For this review, take the finished solid that the model builds, in its own axes (mm). A direction names the side the tool comes from. Round coordinates to 2 decimals unless told otherwise and drop trailing zeros. Write each loop counter-clockwise with the first axis right and the second up, starting at its lowest first coordinate (ties: lowest second). Pieces come first, ordered by that corner, then holes.
from build123d import *

# Parameters (mm, degrees)
SUPPORTOMOTORE_DEPTH     = 30
SCHIZZO2_W               = 58
SCHIZZO2_H               = 39
SUPPORTOESC_DEPTH        = 4
COLONNESUPPORTOESC_REACH = 62.166
SCHIZZO3_R               = 3
SCHIZZO7_W               = 5
SCHIZZO7_H               = 5
SUPPORTIBASEMOTORE_DEPTH = 15
SCHIZZO8_W               = 30
SCHIZZO8_H               = 30
BASEMOTORE_DEPTH         = 2
SCHIZZO9_R               = 1.5
SCHIZZO9_R_2             = 4
FORIAGGANCIOMOTORE_DEPTH = 2
SCHIZZO10_W              = 20
SCHIZZO10_H              = 4
APERTURAFASCETTA_DEPTH   = 4


with BuildPart() as part:
    # Schizzo1 → SupportoMotore (new body)
    with BuildSketch(Plane.XY):
        with BuildLine():
            Line((-2.5, -10.712142643), (-2.5, -15.712142643))
            Line((-2.5, -15.712142643), (-7.5, -15.712142643))
            Line((-7.5, -15.712142643), (-7.5, -8.04673847))
            ThreePointArc((-7.5, -8.04673847), (-10.999946955, -0.034161219), (-7.549834435, 8))
            Line((-7.549834435, 8), (-15.935446939, 8))
            Line((-15.935446939, 8), (-15.935446939, 11))
            Line((-15.935446939, 11), (14.064553061, 11))
            Line((14.064553061, 11), (14.064553061, 8))
            Line((14.064553061, 8), (7.549834435, 8))
            ThreePointArc((7.549834435, 8), (10.999946955, -0.034161219), (7.5, -8.04673847))
            Line((7.5, -8.04673847), (7.5, -15.712142643))
            Line((7.5, -15.712142643), (2.5, -15.712142643))
            Line((2.5, -15.712142643), (2.5, -10.712142643))
            Line((2.5, -10.712142643), (2.5, -8.645808233))
            ThreePointArc((2.5, -8.645808233), (0, 9), (-2.5, -8.645808233))
            Line((-2.5, -8.645808233), (-2.5, -10.712142643))
        make_face()
    extrude(amount=SUPPORTOMOTORE_DEPTH)

    # Schizzo2 → SupportoESC (add)
    with BuildSketch(Plane(origin=(14.064553061, 0, 0), x_dir=(0, 0, -1), z_dir=(1, 0, 0))):
        with Locations((-15, -8.5)):
            Rectangle(SCHIZZO2_W, SCHIZZO2_H)
    extrude(amount=SUPPORTOESC_DEPTH)

    # Schizzo3 → ColonneSupportoESC (add, up to next)
    with BuildSketch(Plane.ZY.offset(-14.064553061), mode=Mode.PRIVATE) as colonnesupportoesc_sk1:
        with Locations(Location((22, -6, 0), (0, 0, 223.019415965))):
            Circle(SCHIZZO3_R)
    colonnesupportoesc_tool1 = extrude(colonnesupportoesc_sk1.sketch, amount=COLONNESUPPORTOESC_REACH, mode=Mode.PRIVATE) - part.part
    # Schizzo3 → ColonneSupportoESC (add, up to next)
    with BuildSketch(Plane.ZY.offset(-14.064553061), mode=Mode.PRIVATE) as colonnesupportoesc_sk2:
        with Locations(Location((8, -6, 0), (0, 0, 223.019415965))):
            Circle(SCHIZZO3_R)
    colonnesupportoesc_tool2 = extrude(colonnesupportoesc_sk2.sketch, amount=COLONNESUPPORTOESC_REACH, mode=Mode.PRIVATE) - part.part
    add(colonnesupportoesc_tool1.solids().sort_by_distance((14.064553, -6, 22))[0])
    add(colonnesupportoesc_tool2.solids().sort_by_distance((14.064553, -6, 8))[0])

    # Schizzo7 → SupportiBaseMotore (add)
    with BuildSketch(Plane(origin=(0, 11, 0), x_dir=(1, 0, 0), z_dir=(0, 1, 0))):
        with Locations((-13.435446939, -27.5)):
            Rectangle(SCHIZZO7_W, SCHIZZO7_H)
        with Locations((11.564553061, -27.5)):
            Rectangle(SCHIZZO7_W, SCHIZZO7_H)
        with Locations((11.564553061, -2.5)):
            Rectangle(SCHIZZO7_W, SCHIZZO7_H)
        with Locations((-13.435446939, -2.5)):
            Rectangle(SCHIZZO7_W, SCHIZZO7_H)
    extrude(amount=SUPPORTIBASEMOTORE_DEPTH)

    # Schizzo8 → BaseMotore (add)
    with BuildSketch(Plane(origin=(0, 26, 0), x_dir=(1, 0, 0), z_dir=(0, 1, 0))):
        with Locations((-0.935446939, -15)):
            Rectangle(SCHIZZO8_W, SCHIZZO8_H)
    extrude(amount=BASEMOTORE_DEPTH)

    # Schizzo9 → ForiAggancioMotore (cut)
    with BuildSketch(Plane(origin=(0, 28, 0), x_dir=(1, 0, 0), z_dir=(0, 1, 0))):
        with Locations(Location((2.623315698, -23.808246618, 0), (0, 0, 270))):
            Circle(SCHIZZO9_R)
        with Locations(Location((-9.743693557, -18.558762637, 0), (0, 0, 270))):
            Circle(SCHIZZO9_R)
        with Locations(Location((-4.494209576, -6.191753382, 0), (0, 0, 270))):
            Circle(SCHIZZO9_R)
        with Locations(Location((7.872799679, -11.441237363, 0), (0, 0, 270))):
            Circle(SCHIZZO9_R)
        with Locations(Location((-0.935446939, -15, 0), (0, 0, 270))):
            Circle(SCHIZZO9_R_2)
    extrude(amount=-FORIAGGANCIOMOTORE_DEPTH, mode=Mode.SUBTRACT)

    # Schizzo10 → AperturaFascetta (cut)
    with BuildSketch(Plane(origin=(18.064553061, 0, 0), x_dir=(0, 0, -1), z_dir=(1, 0, 0))):
        with Locations((-15, 6)):
            Rectangle(SCHIZZO10_W, SCHIZZO10_H)
        with Locations((-15, -23)):
            Rectangle(SCHIZZO10_W, SCHIZZO10_H)
    extrude(amount=-APERTURAFASCETTA_DEPTH, mode=Mode.SUBTRACT)


solid = part.part
(1) We need section A-A, the plane y = 16.5. Give the boundary of the cut face in (x, z).
Geometry check:
outline: (-15.94, 0) - (-10.94, 0) - (-10.94, 5) - (-15.94, 5) - close; (-15.94, 25) - (-10.94, 25) - (-10.94, 30) - (-15.94, 30) - close; (9.06, 0) - (14.06, 0) - (14.06, 5) - (9.06, 5) - close; (9.06, 25) - (14.06, 25) - (14.06, 30) - (9.06, 30) - close
(2) For pin 1 Ø1 at (y, z) = (-9, 4) entering from -X; pin 2 Ø5.5 at (x, z) = (4.5, 11.5) entering from -Y; pin 3 Ø5.5 at (x, z) = (11, 8) entering from -Y, all flat-tipped, find the tip position at first contact; note any pin that passes through.
Geometry check:
pin 1: stops at x = -7.5
pin 2: stops at y = -15.71
pin 3: stops at y = -9
(3) We need section D-D, the plane z = 15. State how many separate pieces and enclosed holes the cut face has, and give its area (3 significant figures).
Geometry check:
separate pieces: 5
enclosed holes: 0
area: 403 mm2
(4) Mouldability with a two-part tool opening along X and no side actions: class faces 1 (the face through (-15.935, 17.9, 25.2)), 2 (the face through (11.56, -8.95, 8.55)), 3 (the face through (16, -21, 15)) as pulls with the +X half, pulls with the -X half, needs draft (parallel to the pull), parting line crosses it, or undercut.
Geometry check:
face 1: pulls with the -X half
face 2: undercut
face 3: needs draft
(5) We need section B-B, the plane z = 27. Give the boundary of the cut face in (x, y).
Geometry check:
outline: (-15.94, 8) - (-7.55, 8) arc R11 ccw to (-7.5, -8.05) - (-7.5, -15.71) - (-2.5, -15.71) - (-2.5, -8.65) arc R9 cw (long way) to (2.5, -8.65) - (2.5, -15.71) - (7.5, -15.71) - (7.5, -8.05) arc R11 ccw to (7.55, 8) - (14.06, 8) - (14.06, -28) - (18.06, -28) - (18.06, 11) - (14.06, 11) - (14.06, 28) - (-15.94, 28) - close; hole (-10.94, 11) - (9.06, 11) - (9.06, 26) - (-10.94, 26) - close
(6) For line 1 along Y through (x, z) = (5, 17); line 2 along Y through (x, z) = (-11.5, 20); line 3 along Y through (x, z) = (16, 21), list the stretches that pass through material, from the lowest coordinate up.
Geometry check:
line 1: y = -15.71 to -7.48, 7.48 to 11, 26 to 28
line 2: y = 8 to 11, 26 to 28
line 3: y = -28 to -25, -21 to 4, 8 to 11
(7) For faces 4 (the face through (-10.935, 18, 3)), 5 (the face through (5, -15.712, 15)), 6 (the face through (-12, 8, 15)), list the 3-axis set-ups (+Z, -Z, +X, -X, +Y, -Y) from which the entire face can be reached by the end or side of a thin tool; tool diameter is ignored.
Geometry check:
face 4: +Z, -Z
face 5: +Z, -Z, -X, -Y
face 6: +Z, -Z, -X
(8) We need section C-C, the plane y = -10. Give the boundary of the cut face in (x, z), and give its area (3 significant figures).
Geometry check:
outline: (-7.5, 0) - (-2.5, 0) - (-2.5, 30) - (-7.5, 30) - close; (2.5, 0) - (7.5, 0) - (7.5, 30) - (2.5, 30) - close; (14.06, -14) - (18.06, -14) - (18.06, 44) - (14.06, 44) - close
area: 532 mm2
